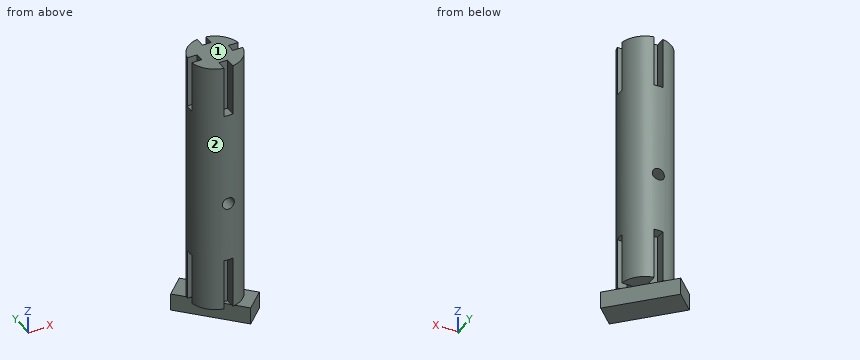
from build123d import *

# Parameters (mm, degrees)
SKETCH1_R                           = 1.5
BOSS_EXTRUDE1_DEPTH                 = 15
SKETCH2_W                           = 0.747320827
SKETCH2_H                           = 0.5
CUT_EXTRUDE1_DEPTH                  = 3
CIRPATTERN1_COUNT                   = 4
MIRROR1_COPY_1_SKETCH_W             = 0.747320827
MIRROR1_COPY_1_SKETCH_H             = 0.5
MIRROR1_COPY_1_DEPTH                = 3
MIRROR1_COPY_2_SKETCH_W             = 0.747320827
MIRROR1_COPY_2_SKETCH_H             = 0.5
MIRROR1_COPY_2_DEPTH                = 3
MIRROR1_COPY_3_SKETCH_W             = 0.747320827
MIRROR1_COPY_3_SKETCH_H             = 0.5
MIRROR1_COPY_3_DEPTH                = 3
BOSS_EXTRUDE5_DEPTH                 = 1
CUT_EXTRUDE2_REACH                  = 17.278
CUT_EXTRUDE2_END_RADIUS             = 1.5
SKETCH7_R                           = 0.35
CUT_EXTRUDE2_DIRECTION_2_REACH      = 17.278
CUT_EXTRUDE2_DIRECTION_2_END_RADIUS = 1.5


with BuildPart() as part:
    # Sketch1 → Boss-Extrude1 (new body)
    with BuildSketch(Plane.XY):
        Circle(SKETCH1_R)
    extrude(amount=BOSS_EXTRUDE1_DEPTH)

    # Sketch2 → Cut-Extrude1 (cut)
    with BuildSketch(Plane(origin=(0, 0, 0), x_dir=(-1, 0, 0), z_dir=(0, 0, -1))):
        with Locations((1.273660414, 0)):
            Rectangle(SKETCH2_W, SKETCH2_H)
    cut_extrude1 = extrude(amount=-CUT_EXTRUDE1_DEPTH, mode=Mode.SUBTRACT)

    # CirPattern1: Cut-Extrude1 ×4 about axis
    cirpattern1_axis = Axis((0, 0, 0), (0, 0, 1))
    for i in range(1, CIRPATTERN1_COUNT):
        add(cut_extrude1.rotate(cirpattern1_axis, i * 360 / CIRPATTERN1_COUNT), mode=Mode.SUBTRACT)

    # Mirror1: Cut-Extrude1 across plane
    add(cut_extrude1.mirror(Plane(origin=(0, 0, 7.5), x_dir=(1, 0, 0), z_dir=(0, 0, -1))), mode=Mode.SUBTRACT)

    # Mirror1 copy 1 sketch → Mirror1 copy 1 (cut)
    with BuildSketch(Plane(origin=(0, 0, 15), x_dir=(0, -1, 0), z_dir=(0, 0, 1))):
        with Locations((1.273660414, 0)):
            Rectangle(MIRROR1_COPY_1_SKETCH_W, MIRROR1_COPY_1_SKETCH_H)
    extrude(amount=-MIRROR1_COPY_1_DEPTH, mode=Mode.SUBTRACT)

    # Mirror1 copy 2 sketch → Mirror1 copy 2 (cut)
    with BuildSketch(Plane.XY.offset(15)):
        with Locations((1.273660414, 0)):
            Rectangle(MIRROR1_COPY_2_SKETCH_W, MIRROR1_COPY_2_SKETCH_H)
    extrude(amount=-MIRROR1_COPY_2_DEPTH, mode=Mode.SUBTRACT)

    # Mirror1 copy 3 sketch → Mirror1 copy 3 (cut)
    with BuildSketch(Plane(origin=(0, 0, 15), x_dir=(0, 1, 0), z_dir=(0, 0, 1))):
        with Locations((1.273660414, 0)):
            Rectangle(MIRROR1_COPY_3_SKETCH_W, MIRROR1_COPY_3_SKETCH_H)
    extrude(amount=-MIRROR1_COPY_3_DEPTH, mode=Mode.SUBTRACT)

    # Sketch6 → Boss-Extrude5 (add)
    with BuildSketch(Plane(origin=(0, 0, 0), x_dir=(-1, 0, 0), z_dir=(0, 0, -1))):
        Polygon((-0.989949494, -2.050609665), (-2.050609665, -0.989949494), (0.989949494, 2.050609665), (2.050609665, 0.989949494), align=None)
    extrude(amount=BOSS_EXTRUDE5_DEPTH)

    # Cut-Extrude2: up to this cylinder (the profile starts inside it)
    cut_extrude2_end = Plane(origin=(0, 0, 6.5), z_dir=(0, 0, -1)) * Cylinder(CUT_EXTRUDE2_END_RADIUS, 38.556, mode=Mode.PRIVATE)
    # Sketch7 → Cut-Extrude2 (cut, up to the surface)
    with BuildSketch(Plane(origin=(0, 0, 0), x_dir=(1, 0, 0), z_dir=(0, 1, 0)), mode=Mode.PRIVATE) as cut_extrude2_sk1:
        with Locations(Location((0, -6.5, 0), (0, 0, 270))):
            Circle(SKETCH7_R)
    cut_extrude2_tool1 = extrude(cut_extrude2_sk1.sketch, amount=-CUT_EXTRUDE2_REACH, mode=Mode.PRIVATE) & cut_extrude2_end
    add(cut_extrude2_tool1.solids().sort_by_distance((0, 0, 6.5))[0], mode=Mode.SUBTRACT)

    # Cut-Extrude2 direction 2: up to this cylinder (the profile starts inside it)
    cut_extrude2_direction_2_end = Plane(origin=(0, 0, 6.5), z_dir=(0, 0, -1)) * Cylinder(CUT_EXTRUDE2_DIRECTION_2_END_RADIUS, 38.556, mode=Mode.PRIVATE)
    # Sketch7 → Cut-Extrude2 direction 2 (cut, up to the surface)
    with BuildSketch(Plane(origin=(0, 0, 0), x_dir=(1, 0, 0), z_dir=(0, 1, 0)), mode=Mode.PRIVATE) as cut_extrude2_direction_2_sk1:
        with Locations(Location((0, -6.5, 0), (0, 0, 270))):
            Circle(SKETCH7_R)
    cut_extrude2_direction_2_tool1 = extrude(cut_extrude2_direction_2_sk1.sketch, amount=CUT_EXTRUDE2_DIRECTION_2_REACH, mode=Mode.PRIVATE) & cut_extrude2_direction_2_end
    add(cut_extrude2_direction_2_tool1.solids().sort_by_distance((0, 0, 6.5))[0], mode=Mode.SUBTRACT)


solid = part.part
For this review, take the finished solid that the model builds, in its own axes (mm). Face numbers are marked on the shaded views. Round coordinates to 2 decimals unless told otherwise and drop trailing zeros. Write each loop counter-clockwise with the first axis right and the second up, starting at its lowest first coordinate (ties: lowest second). Pieces come first, ordered by that corner, then holes. Notation, with made-up numbers: (-3.75, 46.25) -> (4.25, 46.25) arc R15 ccw to (4.25, 60.25) -> close; hole circle Ø10 at (61.5, 51.25). An arc over 180 degrees is marked (long way). Put each result on its own line as item: value.
Q1. The part is to be moulded in two halves that separate along X. For the marked faces 1 and 2, say which applies: released by +X, released by -X, zero draft, split by the parting line, or undercut.
Determined:
face 1: zero draft
face 2: split by the parting line
Q2. Consider section D-D on z = 11.75. State the section outline as (x, y) points, and give its area (3 significant figures).
Determined:
outline: circle Ø3 at (0, 0)
area: 7.07 mm^2
Q3. To check wall thickness, follow L1, parallel to Z at x = -0.75, y = 1.45; L2, parallel to Z at x = 0.8, y = 1.1; L3, parallel to X at y = -0.9, z = 6.5. State the ranges of each line that lie inside material, in increasing order. Write a range as [from, to].
Determined:
L1: z = [-1, 0]
L2: z = [0, 15]
L3: x = [-1.2, -0.35], [0.35, 1.2]
Q4. Consider section B-B on x = 0. State the section outline as (y, z) points.
Determined:
outline: (-1.5, 3) -> (-0.9, 3) -> (-0.9, 0) -> (-1.06, 0) -> (-1.06, -1) -> (1.06, -1) -> (1.06, 0) -> (0.9, 0) -> (0.9, 3) -> (1.5, 3) -> (1.5, 6.15) -> (-1.5, 6.15) -> close; (-1.5, 6.85) -> (1.5, 6.85) -> (1.5, 12) -> (0.9, 12) -> (0.9, 15) -> (-0.9, 15) -> (-0.9, 12) -> (-1.5, 12) -> close
Q5. Consider section A-A on z = 0.25. State the section outline as (x, y) points, and give its area (3 significant figures).
Determined:
outline: (-1.48, -0.25) arc R1.5 ccw to (-0.25, -1.48) -> (-0.25, -0.9) -> (0.25, -0.9) -> (0.25, -1.48) arc R1.5 ccw to (1.48, -0.25) -> (0.9, -0.25) -> (0.9, 0.25) -> (1.48, 0.25) arc R1.5 ccw to (0.25, 1.48) -> (0.25, 0.9) -> (-0.25, 0.9) -> (-0.25, 1.48) arc R1.5 ccw to (-1.48, 0.25) -> (-0.9, 0.25) -> (-0.9, -0.25) -> close
area: 5.88 mm^2
Q6. Clearance check with flat-ended pins moving along their axes: pin 1 Ø0.5 at (y, z) = (1, 2) entering from -X; pin 2 Ø0.5 at (x, z) = (1, 2) entering from -Y; pin 3 Ø0.5 at (y, z) = (-1, 13.5) entering from +X. State where each tip first meets the part, or that it passes through.
Determined:
pin 1: stops at x = -1.3
pin 2: stops at y = -1.3
pin 3: stops at x = 1.3
Q7. Consider section C-C on x = -1.7. State the section outline as (y, z) points.
Determined:
outline: (0.64, -1) -> (1.34, -1) -> (1.34, 0) -> (0.64, 0) -> close
